Input: part model. Units: mm. Frame: model coordinates. A direction names the side the tool comes from. Give positions to 0.01 mm unless a question says otherwise; leave off trailing zeros. Loops run counter-clockwise (first coordinate to the right, second up) from the corner with the lowest first, then second, coordinate; pieces in that order, holes last. Notation, with made-up numbers: (71, 56) -> (114, 56) arc R18 ccw to (114, 77) -> close; hole circle Ø4 at (87.25, 68.5). An arc over 180 degrees is marked (long way). Answer as a JSON object with one key per item and string values.
```python
from build123d import *

# Parameters (mm, degrees)
EXTRUDE_THIN1_DEPTH = 20
SKETCH2_W           = 30
SKETCH2_H           = 20
CUT_EXTRUDE1_DEPTH  = 71
SKETCH3_R           = 6.1
CUT_EXTRUDE2_DEPTH  = 69.767724988
FILLET1_R           = 12


with BuildPart() as part:
    # Sketch1 → Extrude-Thin1 (new, symmetric)
    with BuildSketch(Plane.XY):
        Polygon((-60, 0), (-30, 0), (-30, 9), (-25.5, 9), (-25.5, 18), (-21, 18), (-21, 27), (0, 27), (0, 30), (-24, 30), (-24, 21), (-28.5, 21), (-28.5, 12), (-33, 12), (-33, 3), (-60, 3), align=None)
    extrude_thin1 = extrude(amount=EXTRUDE_THIN1_DEPTH, both=True)

    # Mirror1: Extrude-Thin1 across plane
    add(extrude_thin1.mirror(Plane(origin=(0, 30, -20), x_dir=(0, 0, 1), z_dir=(-1, 0, 0))))

    # Sketch2 → Cut-Extrude1 (cut, through all)
    with BuildSketch(Plane(origin=(0, 30, 0), x_dir=(1, 0, 0), z_dir=(0, 1, 0))):
        Rectangle(SKETCH2_W, SKETCH2_H)
    extrude(amount=-CUT_EXTRUDE1_DEPTH, mode=Mode.SUBTRACT)

    # Sketch3 → Cut-Extrude2 (cut, through all)
    with BuildSketch(Plane(origin=(0, 3, 0), x_dir=(1, 0, 0), z_dir=(0, 1, 0))):
        with Locations(Location((-45, 0, 0), (0, 0, 270))):
            Circle(SKETCH3_R)
    cut_extrude2 = extrude(amount=-CUT_EXTRUDE2_DEPTH, mode=Mode.SUBTRACT)

    # Mirror2: Cut-Extrude2 across plane
    add(cut_extrude2.mirror(Plane(origin=(0, 0, 0), x_dir=(0, 0, 1), z_dir=(1, 0, 0))), mode=Mode.SUBTRACT)

    # Fillet1
    fillet1_edges = [part.edges().sort_by_distance(p)[0] for p in [
        (-60, 1.5, 20),
        (-60, 1.5, -20),
        (60, 1.5, -20),
        (60, 1.5, 20),
    ]]
    fillet(fillet1_edges, radius=FILLET1_R)


solid = part.part
```
Q1. Access query for faces 1 (the flat face through (15, 29, 0)), 2 (the flat face through (-21, 22, 0)), 3 (the flat face through (0, 30, 14)). Directions: +Z, -Z, +X, -X, +Y, -Y. A direction counts if a zero-diameter tool reaches every point of the face in a straight line with its end or side. Return the directions, or none.
Evaluation:
{"face 1": "+Y, -Y", "face 2": "+Z, -Z, -Y", "face 3": "+Z, -Z, +X, -X, +Y"}
Q2. Draft query along X for faces 4 (the cylindrical face through (56.58, 1.48, 16.39)), 5 (the flat face through (30, 4, 0)), 6 (the cylindrical face through (39.856, 1.521, 3.279)), 7 (the flat face through (-49, 3, 5)). Return one class per face: +X half, -X half, draft (parallel to the pull), parting line (faces both ways), or undercut.
Evaluation:
{"face 4": "+X half", "face 5": "undercut", "face 6": "undercut", "face 7": "draft"}
Q3. Section B-B, the plane y = 24.5. Return the cut outline in (x, z), then the cut area to 3 significant figures.
Evaluation:
{"outline": "(-24, -20) -> (-21, -20) -> (-21, 20) -> (-24, 20) -> close; (21, -20) -> (24, -20) -> (24, 20) -> (21, 20) -> close", "area": "240 mm2"}
Q4. Ray query, line 1 along X through (y, z) = (0.7, 0); line 2 along X through (y, z) = (14.25, -18); line 3 along X through (y, z) = (9.25, -17). Return the intervals inside material, ascending.
Evaluation:
{"line 1": "x = -60 to -51.1, -38.9 to -30, 30 to 38.9, 51.1 to 60", "line 2": "x = -28.5 to -25.5, 25.5 to 28.5", "line 3": "x = -33 to -25.5, 25.5 to 33"}
Q5. Section A-A, the plane x = 45. Return the cut outline in (y, z).
Evaluation:
{"outline": "(0, -20) -> (3, -20) -> (3, -6.1) -> (0, -6.1) -> close; (0, 6.1) -> (3, 6.1) -> (3, 20) -> (0, 20) -> close"}
Q6. Section C-C, the plane z = 13.5. Return the cut outline in (x, y).
Evaluation:
{"outline": "(-58.67, 0) -> (-30, 0) -> (-30, 9) -> (-25.5, 9) -> (-25.5, 18) -> (-21, 18) -> (-21, 27) -> (21, 27) -> (21, 18) -> (25.5, 18) -> (25.5, 9) -> (30, 9) -> (30, 0) -> (58.67, 0) -> (58.67, 3) -> (33, 3) -> (33, 12) -> (28.5, 12) -> (28.5, 21) -> (24, 21) -> (24, 30) -> (-24, 30) -> (-24, 21) -> (-28.5, 21) -> (-28.5, 12) -> (-33, 12) -> (-33, 3) -> (-58.67, 3) -> close"}
Q7. Pin query (flat end, axial travel): pin 1 (4.5 mm diameter, centred on y = 14, z = -8, fed in from +X); pin 2 (1.3 mm diameter, centred on x = -23, z = -8.5, fed in from -Y); pin 3 (1.5 mm diameter, centred on y = 28, z = -4, fed in from +X); pin 4 (12 mm diameter, centred on x = 14.5, y = 16, fed in from +Z). Return the tip coordinate at first contact, or that it passes through.
Evaluation:
{"pin 1": "stops at x = 33", "pin 2": "stops at y = 18", "pin 3": "stops at x = 24", "pin 4": "passes through"}
Q8. Section D-D, the plane z = 0. Give the number of separate pieces and of enclosed holes in the cut face, then the cut area to 3 significant figures.
Evaluation:
{"separate pieces": "4", "enclosed holes": "0", "area": "359 mm2"}
